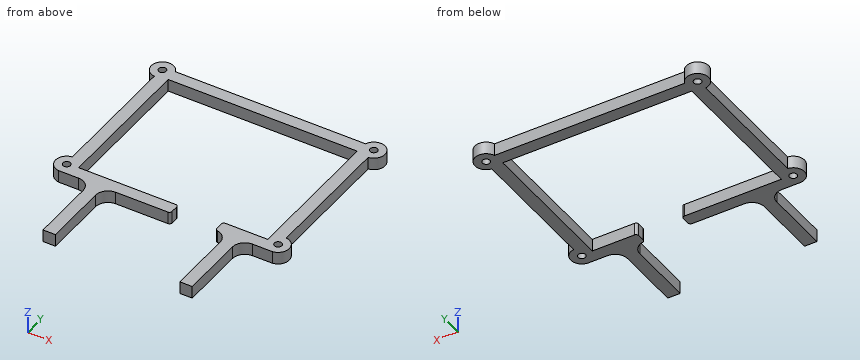
from build123d import *

# Parameters (mm, degrees)
F0_W      = 86
F0_H      = 68
F1_DEPTH  = 5
F2_W      = 76
F2_H      = 58
F3_DEPTH  = 5
F4_W      = 18
F4_H      = 5
F5_DEPTH  = 5
F6_R      = 4.5
F7_DEPTH  = 5
F8_R      = 1.5
F9_DEPTH  = 5
F10_R     = 1
F11_W     = 5
F11_H     = 5
F12_DEPTH = 31
F13_R     = 5


with BuildPart() as f1:
    # F0 (on Top) → F1 (new body)
    with BuildSketch(Plane.XY):
        Rectangle(F0_W, F0_H)
    extrude(amount=F1_DEPTH)

    # F2 (on face) → F3 (cut, through all)
    with BuildSketch(Plane.XY.offset(5)):
        Rectangle(F2_W, F2_H)
    extrude(amount=-F3_DEPTH, mode=Mode.SUBTRACT)

    # F4 (on face) → F5 (cut, through all)
    with BuildSketch(Plane.XY.offset(5)):
        with Locations((11, -31.5)):
            Rectangle(F4_W, F4_H)
    extrude(amount=-F5_DEPTH, mode=Mode.SUBTRACT)

    # F6 (on face) → F7 (join)
    with BuildSketch(Plane.XY.offset(5)):
        with Locations((-42.5, 32.5)):
            Circle(F6_R)
        with Locations((42.5, 32.5)):
            Circle(F6_R)
        with Locations((-42.5, -29.5)):
            Circle(F6_R)
        with Locations((42.5, -29.5)):
            Circle(F6_R)
    extrude(amount=-F7_DEPTH)

    # F8 (on face) → F9 (cut, through all)
    with BuildSketch(Plane.XY.offset(5)):
        with Locations((-42.5, 32.5)):
            Circle(F8_R)
        with Locations((-42.5, -29.5)):
            Circle(F8_R)
        with Locations((42.5, -29.5)):
            Circle(F8_R)
        with Locations((42.5, 32.5)):
            Circle(F8_R)
    extrude(amount=-F9_DEPTH, mode=Mode.SUBTRACT)

    # F10
    f10_edges = [f1.edges().sort_by_distance(p)[0] for p in [
        (20, -29, 2.5),
        (20, -34, 2.5),
        (2, -29, 2.5),
        (2, -34, 2.5),
    ]]
    fillet(f10_edges, radius=F10_R)

    # F11 (on face) → F12 (join)
    with BuildSketch(Plane.XZ.offset(34)):
        with Locations((-27.5, 2.5)):
            Rectangle(F11_W, F11_H)
        with Locations((27.5, 2.5)):
            Rectangle(F11_W, F11_H)
    extrude(amount=F12_DEPTH)

    # F13
    f13_edges = [f1.edges().sort_by_distance(p)[0] for p in [
        (25, -34, 2.5),
        (-25, -34, 2.5),
        (30, -34, 2.5),
        (-30, -34, 2.5),
    ]]
    fillet(f13_edges, radius=F13_R)


solid = f1.part
Read the model definition and answer for the solid it produces. Units are mm, in the model's axes. Coordinates: 2 decimals unless noted, no trailing zeros. Write each loop counter-clockwise with the first axis right and the second up, starting at its lowest first coordinate (ties: lowest second). Pieces come first, ordered by that corner, then holes. Notation, with made-up numbers: (43, -38) -> (52, -38) arc R17 cw to (52, -6) -> close; hole circle Ø2 at (61.25, 78). An arc over 180 degrees is marked (long way). Return JSON: item names as keys, results as strings.
(1) The part is cut by section A-A on y = 5.5. Give the vertices of the cut face in (x, z), then the cut area to 3 significant figures.
Answers below:
{"outline": "(-43, 0) -> (-38, 0) -> (-38, 5) -> (-43, 5) -> close; (38, 0) -> (43, 0) -> (43, 5) -> (38, 5) -> close", "area": "50.0 mm^2"}
(2) Consider line 1 along Y through (x, z) = (42.5, 1); line 2 along X through (y, z) = (-51.5, 1.15); line 3 along X through (y, z) = (26.5, 0.95). Determine where each line is inside the solid, lowest interval first. Write a range as from..to.
Answers below:
{"line 1": "-34..-31, -28..31, 34..37", "line 2": "-30..-25, 25..30", "line 3": "-43..-38, 38..43"}
(3) Each of these flat-tipped pins is pushed along its axis until it touches: P1, Ø1.5, axis at y = 5.5, z = 2.5, coming from the -X side; P2, Ø2.5, axis at x = -42.5, y = 32.5, coming from the -Z side; P3, Ø2, axis at y = -41.5, z = 2, coming from the -X side; P4, Ø1.5, axis at y = -5.5, z = 2, coming from the +X side. Where does it stop, or does it pass through?
Answers below:
{"P1": "x = -43", "P2": "through", "P3": "x = -30", "P4": "x = 43"}
(4) The part is cut by section B-B on y = 32.5. Give the vertices of the cut face in (x, z).
Answers below:
{"outline": "(-47, 0) -> (-44, 0) -> (-44, 5) -> (-47, 5) -> close; (-41, 0) -> (41, 0) -> (41, 5) -> (-41, 5) -> close; (44, 0) -> (47, 0) -> (47, 5) -> (44, 5) -> close"}
